Part model, mm, in its own coordinate system. Face numbers are marked on the shaded views. Coordinates: 2 decimals unless noted, no trailing zeros. Order: outer loops, then holes, each group sorted by start corner. A loop starts at its lowest first (then second) coordinate and runs counter-clockwise, first axis right, second up.
1) Wall check: L1, parallel to Y at x = -4.5, z = 6.25; L2, parallel to X at y = 1.5, z = 0; L3, parallel to Z at x = -0.25, y = 5. Give the ranges that are in metal, low to high.
2) Cut at C-C (y = 6.75). List the corners of the cut face in (x, z), and give its area (3 significant figures).
3) Cut at D-D (z = 3). List the corners of the cut face in (x, y).
4) Cut at A-A (z = 0). List the corners of the cut face in (x, y), and give its area (3 significant figures).
5) Cut at B-B (x = 0). List the corners of the cut face in (y, z), and give its area (3 significant figures).
6) Mould opens along Y. For the marked faces 1, 2, 3 and 4 say: +Y half, -Y half, draft (parallel to the pull), parting line (faces both ways), or undercut.
7) Pin check, flat tips, straight feed: pin 1 Ø4 at (x, y) = (2, 4) entering from -Z; pin 2 Ø4 at (x, z) = (-2.5, -1) entering from -Y; pin 3 Ø2 at (y, z) = (4, -1) entering from -X; pin 4 Ø3 at (x, z) = (0, 0) entering from -Y. Stop position of each tip, or through.
```python
from build123d import *

# Parameters (mm, degrees)
SKIZZE1_R                       = 9
SKIZZE1_R_2                     = 6
AUFSATZ_LINEAR_AUSTRAGEN1_DEPTH = 1
SKIZZE1_3_R                     = 6
SKIZZE1_3_R_2                   = 2
AUFSATZ_LINEAR_AUSTRAGEN2_DEPTH = 6.5
SKIZZE2_R                       = 9
SKIZZE2_R_2                     = 2
AUFSATZ_LINEAR_AUSTRAGEN3_DEPTH = 1


with BuildPart() as part:
    # Skizze1 → Aufsatz-Linear austragen1 (new body)
    with BuildSketch(Plane(origin=(0, 0, 0), x_dir=(1, 0, 0), z_dir=(0, 1, 0))):
        with Locations(Location((0, 0, 0), (0, 0, 270))):
            Circle(SKIZZE1_R)
        with Locations(Location((0, 0, 0), (0, 0, 270))):
            Circle(SKIZZE1_R_2, mode=Mode.SUBTRACT)
    extrude(amount=AUFSATZ_LINEAR_AUSTRAGEN1_DEPTH)

    # Skizze1_3 → Aufsatz-Linear austragen2 (add)
    with BuildSketch(Plane(origin=(0, 0, 0), x_dir=(1, 0, 0), z_dir=(0, 1, 0))):
        with Locations(Location((0, 0, 0), (0, 0, 90))):
            Circle(SKIZZE1_3_R)
        with Locations(Location((0, 0, 0), (0, 0, 90))):
            Circle(SKIZZE1_3_R_2, mode=Mode.SUBTRACT)
    extrude(amount=AUFSATZ_LINEAR_AUSTRAGEN2_DEPTH)

    # Skizze2 → Aufsatz-Linear austragen3 (add)
    with BuildSketch(Plane(origin=(0, 6.5, 0), x_dir=(1, 0, 0), z_dir=(0, 1, 0))):
        with Locations(Location((0, 0, 0), (0, 0, 270))):
            Circle(SKIZZE2_R)
        with Locations(Location((0, 0, 0), (0, 0, 90))):
            Circle(SKIZZE2_R_2, mode=Mode.SUBTRACT)
    extrude(amount=AUFSATZ_LINEAR_AUSTRAGEN3_DEPTH)


solid = part.part
```
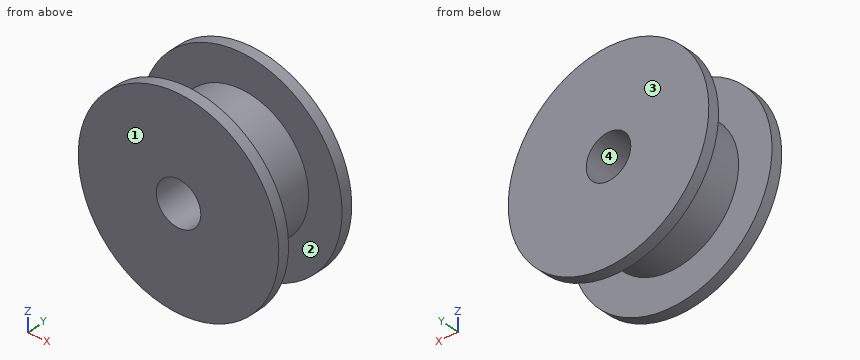
Geometry check:
1. L1: y = 0 to 1, 6.5 to 7.5
1. L2: x = -6 to -2, 2 to 6
1. L3: z = -5.99 to -1.98, 1.98 to 5.99
2. outline: circle Ø18 at (0, 0); hole circle Ø4 at (0, 0)
2. area: 242 mm2
3. outline: (-8.49, 0) - (8.49, 0) - (8.49, 1) - (5.2, 1) - (5.2, 6.5) - (8.49, 6.5) - (8.49, 7.5) - (-8.49, 7.5) - (-8.49, 6.5) - (-5.2, 6.5) - (-5.2, 1) - (-8.49, 1) - close
4. outline: (-9, 0) - (-2, 0) - (-2, 7.5) - (-9, 7.5) - (-9, 6.5) - (-6, 6.5) - (-6, 1) - (-9, 1) - close; (2, 0) - (9, 0) - (9, 1) - (6, 1) - (6, 6.5) - (9, 6.5) - (9, 7.5) - (2, 7.5) - close
4. area: 72.0 mm2
5. outline: (0, -9) - (1, -9) - (1, -6) - (6.5, -6) - (6.5, -9) - (7.5, -9) - (7.5, -2) - (0, -2) - close; (0, 2) - (7.5, 2) - (7.5, 9) - (6.5, 9) - (6.5, 6) - (1, 6) - (1, 9) - (0, 9) - close
5. area: 72.0 mm2
6. face 1: -Y half
6. face 2: undercut
6. face 3: +Y half
6. face 4: draft
7. pin 1: stops at z = -6
7. pin 2: stops at y = 0
7. pin 3: stops at x = -6
7. pin 4: passes through
